Can you work these out from the drawing? Everything is in mm from the part's minimum corner. Round coordinates to 2 decimals unless told otherwise and drop trailing zeros. Loops run counter-clockwise (first coordinate to the right, second up) from the corner with the lowest first, then second, coordinate; pieces in that order, holes last. Notation, with made-up numbers: (68.5, 2.25) - (104.5, 2.25) arc R27 cw to (104.5, 22.25) - close; hole circle Ø8 at (-14.75, 41). An arc over 180 degrees is marked (long way). Put each result on its own line as item: value. Start each with the question number.
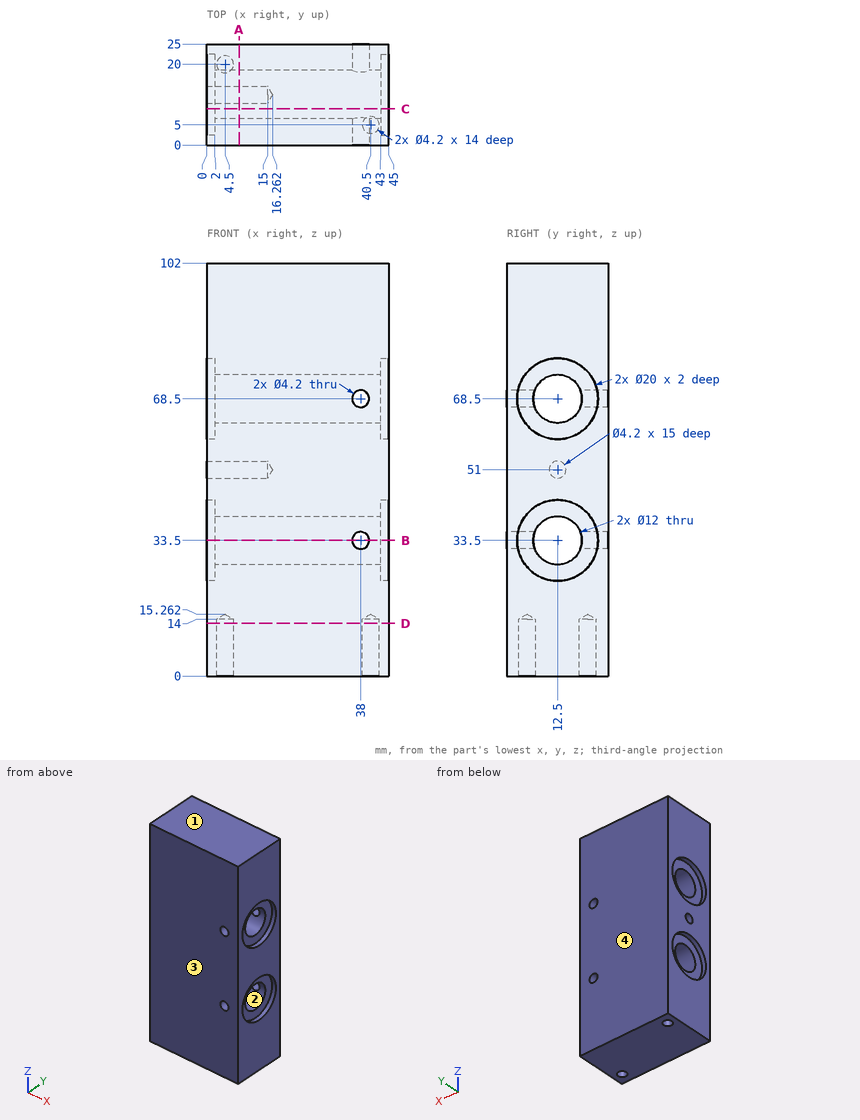
Item 1: I need wall thicknesses on line 1 (Z direction, x = 37.5, y = 8.25) (1 decimal); line 2 (Y direction, x = 0.9, z = 33.5); line 3 (Z direction, x = 22, y = 17.5). Which ranges of each line are inside material? Lowest first, please. Write a range as from..to.
Item 2: Thinking about a two-plate mould opening in Y: for the marked faces 1, 2, 3 and 4, which applies, released by +Y, released by -Y, zero draft, split by the parting line, or undercut?
Item 3: Will these pins go through, and if not, where does the flat tip stop? P1, Ø10, axis at y = 16.5, z = 69, coming from the +X side; P2, Ø2.5, axis at y = 12.5, z = 51, coming from the -X side; P3, Ø2.5, axis at x = 38, z = 68.5, coming from the +Y side; P4, Ø6, axis at y = 17, z = 37.5, coming from the -X side.
Item 4: Suppose I cut it at B-B, the plane z = 33.5. List the corners of the cut face in (x, y) for me.
Item 5: Suppose I cut it at A-A, the plane x = 8. List the corners of the cut face in (y, z) for me.
Item 6: Suppose I cut it at D-D, the plane z = 13. List the corners of the cut face in (x, y) for me, then the cut area to 3 significant figures.
Item 7: Suppose I cut it at C-C, the plane y = 9. List the corners of the cut face in (x, z) for me, then the cut area to 3 significant figures.
Numbers:
1. line 1: 0..29.3, 37.7..64.3, 72.7..102
1. line 2: 0..2.5, 22.5..25
1. line 3: 0..30.18, 36.82..65.18, 71.82..102
2. face 1: zero draft
2. face 2: undercut
2. face 3: released by -Y
2. face 4: released by +Y
3. P1: x = 43
3. P2: x = 15.51
3. P3: through
3. P4: x = 2
4. outline: (0, 0) - (35.9, 0) - (35.9, 6.5) - (2, 6.5) - (2, 2.5) - (0, 2.5) - close; (0, 22.5) - (2, 22.5) - (2, 18.5) - (35.9, 18.5) - (35.9, 25) - (0, 25) - close; (40.1, 0) - (45, 0) - (45, 2.5) - (43, 2.5) - (43, 6.5) - (40.1, 6.5) - close; (40.1, 18.5) - (43, 18.5) - (43, 22.5) - (45, 22.5) - (45, 25) - (40.1, 25) - close
5. outline: (0, 0) - (25, 0) - (25, 102) - (0, 102) - close; hole circle Ø12 at (12.5, 33.5); hole circle Ø12 at (12.5, 68.5); hole circle Ø4.2 at (12.5, 51)
6. outline: (0, 0) - (45, 0) - (45, 25) - (0, 25) - close; hole circle Ø4.2 at (4.5, 20); hole circle Ø4.2 at (40.5, 5)
6. area: 1,100 mm^2
7. outline: (0, 0) - (45, 0) - (45, 24.13) - (43, 24.13) - (43, 28.63) - (2, 28.63) - (2, 24.13) - (0, 24.13) - close; (0, 42.87) - (2, 42.87) - (2, 38.37) - (43, 38.37) - (43, 42.87) - (45, 42.87) - (45, 59.13) - (43, 59.13) - (43, 63.63) - (2, 63.63) - (2, 59.13) - (0, 59.13) - close; (0, 77.87) - (2, 77.87) - (2, 73.37) - (43, 73.37) - (43, 77.87) - (45, 77.87) - (45, 102) - (0, 102) - close
7. area: 3,640 mm^2
